from build123d import *

# Parameters (mm, degrees)
ESQUISSE1_R                  = 10
BOSS_EXTRU_1_DEPTH           = 2
D_GAGEMENT_M21_D             = 2.4
R_P_TITION_CIRCULAIRE1_COUNT = 4
ESQUISSE4_R                  = 3
BOSS_EXTRU_2_DEPTH           = 10
ESQUISSE5_W                  = 6
ESQUISSE5_H                  = 1.22
ENL_V_MAT_EXTRU_1_DEPTH      = 10


with BuildPart() as part:
    # Esquisse1 → Boss.-Extru.1 (new body)
    with BuildSketch(Plane.XY):
        Circle(ESQUISSE1_R)
    extrude(amount=BOSS_EXTRU_1_DEPTH)

    # Dégagement M21 (through all)
    with Locations(Plane(origin=(-0.098042357, 7.745346196, 2), x_dir=(1, 0, 0), z_dir=(0, 0, 1))):
        with Locations((0, 0)):
            d_gagement_m21 = Hole(D_GAGEMENT_M21_D / 2)

    # Répétition circulaire1: Dégagement M21 ×4 about axis
    r_p_tition_circulaire1_axis = Axis((0.001432437, -0.113162526, 0), (0, 0, 1))
    for i in range(1, R_P_TITION_CIRCULAIRE1_COUNT):
        add(d_gagement_m21.rotate(r_p_tition_circulaire1_axis, i * 360 / R_P_TITION_CIRCULAIRE1_COUNT), mode=Mode.SUBTRACT)

    # Esquisse4 → Boss.-Extru.2 (add)
    with BuildSketch(Plane.XY.offset(2)):
        Circle(ESQUISSE4_R)
    extrude(amount=BOSS_EXTRU_2_DEPTH)

    # Esquisse5 → Enlèv. mat.-Extru.1 (cut)
    with BuildSketch(Plane.XY.offset(12)):
        with Locations((0, 2.39)):
            Rectangle(ESQUISSE5_W, ESQUISSE5_H)
    extrude(amount=-ENL_V_MAT_EXTRU_1_DEPTH, mode=Mode.SUBTRACT)


solid = part.part
For this review, take the finished solid that the model builds, in its own axes (mm). A direction names the side the tool comes from. Round coordinates to 2 decimals unless told otherwise and drop trailing zeros. Write each loop counter-clockwise with the first axis right and the second up, starting at its lowest first coordinate (ties: lowest second). Pieces come first, ordered by that corner, then holes. Notation, with made-up numbers: M -7,37 L 4,37 A13 ccw 4,56 Z; hole C -5.75,-38 d11. An arc over 180 degrees is marked long. Write item = value, one per line. Start each with the question number.
(1) We need section A-A (x = 0). Give the boundary of the cut face in (y, z), then the cut area to 3 significant figures.
(2) Clearance check with flat-ended pins moving along their axes: pin 1 Ø1.4 at (x, z) = (-1, 7) entering from +Y; pin 2 Ø4 at (x, y) = (-6.5, -8) entering from +Z. State where each tip first meets the part, or that it passes through.
(3) We need section C-C (z = 7). Give the boundary of the cut face in (x, y), then the cut area to 3 significant figures.
(4) For line 1 along Z through (x, y) = (-5.5, -2.25); line 2 along Y through (x, z) = (-2, 2.5); line 3 along X through (y, z) = (1.25, 4.75), list the stretches that pass through material, from the lowest coordinate up.
(5) The part is to be moulded in two halves that separate along X. For faces 3 (the face through (9.05, -0.17, 0.99)), 4 (the face through (0.058, 8.935, 0.986)), 5 (the face through (-2.17, -9.76, 0.99)), 6 (the face through (0, 1.78, 7)), say which applies: +X half, -X half, draft (parallel to the pull), parting line (faces both ways), or undercut.
(6) For faces 1 (the face through (0, -3, 7)), 2 (the face through (-0.06, -9.16, 0.99)), list the 3-axis set-ups (+Z, -Z, +X, -X, +Y, -Y) from which the entire face can be reached by the end or side of a thin tool; tool diameter is ignored.
(7) We need section D-D (y = -2.75). Give the boundary of the cut face in (x, z).
(8) We need section B-B (y = 0). Give the boundary of the cut face in (x, z).
Results found:
q1.outline = M -10,0 L -9.17,0 L -9.17,2 L -10,2 Z; M -6.78,0 L 6.55,0 L 6.55,2 L 1.78,2 L 1.78,12 L -3,12 L -3,2 L -6.78,2 Z; M 8.94,0 L 10,0 L 10,2 L 8.94,2 Z
q1.area = 78.2 mm²
q2.pin_1 = 1.78
q2.pin_2 = 2
q3.outline = M -2.41,1.78 A3 ccw long 2.41,1.78 Z
q3.area = 24.2 mm²
q4.line_1 = 0 to 2
q4.line_2 = -2.24 to 1.78
q4.line_3 = -2.73 to 2.73
q5.face_3 = undercut
q5.face_4 = undercut
q5.face_5 = parting line
q5.face_6 = draft
q6.face_1 = +Z
q6.face_2 = +Z, -Z
q7.outline = M -9.61,0 L 9.61,0 L 9.61,2 L 1.2,2 L 1.2,12 L -1.2,12 L -1.2,2 L -9.61,2 Z
q8.outline = M -10,0 L -9.04,0 L -9.04,2 L -10,2 Z; M -6.68,0 L 6.66,0 L 6.66,2 L 3,2 L 3,12 L -3,12 L -3,2 L -6.68,2 Z; M 9.06,0 L 10,0 L 10,2 L 9.06,2 Z
